```python
from build123d import *

# Parameters (mm, degrees)
ESQUISSE1_R        = 115
ESQUISSE1_R_2      = 85
ESQUISSE1_R_3      = 1.5
ESQUISSE1_W        = 5
ESQUISSE1_H        = 5
BOSS_EXTRU_1_DEPTH = 5


with BuildPart() as part:
    # Esquisse1 → Boss.-Extru.1 (new body)
    with BuildSketch(Plane.XY):
        Circle(ESQUISSE1_R)
        Circle(ESQUISSE1_R_2, mode=Mode.SUBTRACT)
        with Locations((-100, 0)):
            Circle(ESQUISSE1_R_3, mode=Mode.SUBTRACT)
        with Locations((0, 100)):
            Circle(ESQUISSE1_R_3, mode=Mode.SUBTRACT)
        with Locations((100, 0)):
            Circle(ESQUISSE1_R_3, mode=Mode.SUBTRACT)
        with Locations((0, -100)):
            Circle(ESQUISSE1_R_3, mode=Mode.SUBTRACT)
        with Locations((-100, -7.5)):
            Rectangle(ESQUISSE1_W, ESQUISSE1_H, mode=Mode.SUBTRACT)
        with Locations((-100, 7.5)):
            Rectangle(ESQUISSE1_W, ESQUISSE1_H, mode=Mode.SUBTRACT)
        with Locations((-7.5, 100)):
            Rectangle(ESQUISSE1_W, ESQUISSE1_H, mode=Mode.SUBTRACT)
        with Locations((7.5, 100)):
            Rectangle(ESQUISSE1_W, ESQUISSE1_H, mode=Mode.SUBTRACT)
        with Locations((100, 7.5)):
            Rectangle(ESQUISSE1_W, ESQUISSE1_H, mode=Mode.SUBTRACT)
        with Locations((100, -7.5)):
            Rectangle(ESQUISSE1_W, ESQUISSE1_H, mode=Mode.SUBTRACT)
        with Locations((7.5, -100)):
            Rectangle(ESQUISSE1_W, ESQUISSE1_H, mode=Mode.SUBTRACT)
        with Locations((-7.5, -100)):
            Rectangle(ESQUISSE1_W, ESQUISSE1_H, mode=Mode.SUBTRACT)
    extrude(amount=BOSS_EXTRU_1_DEPTH)


solid = part.part
```
Read the model definition and answer for the solid it produces. Units are mm, in the model's axes. Give positions to 0.01 mm unless a question says otherwise; leave off trailing zeros. Order: outer loops, then holes, each group sorted by start corner. A loop starts at its lowest first (then second) coordinate and runs counter-clockwise, first axis right, second up. Notation, with made-up numbers: (-5, 80.5) -> (34, 80.5) arc R34 cw to (34, 110.5) -> close; hole circle Ø3 at (82.25, 88). An arc over 180 degrees is marked (long way). Write item = value, one per line.
1. A cutting plane is placed at A-A, the plane x = -80. Write down the section's boundary in (y, z).
Numbers:
outline = (-82.61, 0) -> (-28.72, 0) -> (-28.72, 5) -> (-82.61, 5) -> close; (28.72, 0) -> (82.61, 0) -> (82.61, 5) -> (28.72, 5) -> close
2. The mould has two halves that part along Y. Classify faces 1 (the face through (100, 10, 2)), 2 (the face through (-97.5, -8, 2)), 3 (the face through (-69, -51, 0)): +Y half, -Y half, draft (parallel to the pull), parting line (faces both ways), or undercut.
Numbers:
face_1 = undercut
face_2 = undercut
face_3 = draft
3. Given pin 1 (1.5 mm diameter, centred on x = -100.5, z = 1.5, fed in from -Y); pin 2 (1.5 mm diameter, centred on x = 100.5, z = 1.5, fed in from +Y); pin 3 (2 mm diameter, centred on y = 47, z = 0.5, fed in from -X), each flat-ended and moving along its own axis, determine where each tip first touches the part or whether it passes through.
Numbers:
pin_1 = -57.23
pin_2 = 57.23
pin_3 = -105.4
4. A cutting plane is placed at C-C, the plane z = 3.55. Count the separate pieces of the cut face and the enclosed holes in it, and give its area (3 significant figures).
Numbers:
separate_pieces = 1
enclosed_holes = 13
area = 18,600 mm²
5. Straight lines are drawn through the part: line 1 along Y through (x, z) = (0, 2.55); line 2 along Y through (x, z) = (100, 3.2). For each, find the intervals that lie inside material, in ascending order.
Numbers:
line_1 = -115 to -101.5, -98.5 to -85, 85 to 98.5, 101.5 to 115
line_2 = -56.79 to -10, -5 to -1.5, 1.5 to 5, 10 to 56.79
6. A cutting plane is placed at B-B, the plane y = -58.5. Write down the section's boundary in (x, z).
Numbers:
outline = (-99.01, 0) -> (-61.67, 0) -> (-61.67, 5) -> (-99.01, 5) -> close; (61.67, 0) -> (99.01, 0) -> (99.01, 5) -> (61.67, 5) -> close
